```python
from build123d import *

# Parameters (mm, degrees)
SCHIZZO1_W                   = 63.34
SCHIZZO1_H                   = 103.98
ESTRUSIONE_ESTRUSIONE1_DEPTH = 4
SCHIZZO2_W                   = 63.34
SCHIZZO2_H                   = 103.98
SCHIZZO2_W_2                 = 53.34
SCHIZZO2_H_2                 = 93.98
ESTRUSIONE_ESTRUSIONE2_DEPTH = 35
FORO_PER_VITE_M2_1_D         = 2.4
SCHIZZO5_W                   = 33.34
SCHIZZO5_H                   = 15
TAGLIO_ESTRUSIONE1_DEPTH     = 126.106755432
TAGLIO_ESTRUSIONE2_DEPTH     = 132.87260726
RACCORDO1_R                  = 4


with BuildPart() as part:
    # Schizzo1 → Estrusione-Estrusione1 (new body)
    with BuildSketch(Plane(origin=(0, 0, 0), x_dir=(1, 0, 0), z_dir=(0, 1, 0))):
        with Locations((34.160538922, 55.414491018)):
            Rectangle(SCHIZZO1_W, SCHIZZO1_H)
    extrude(amount=ESTRUSIONE_ESTRUSIONE1_DEPTH)

    # Schizzo2 → Estrusione-Estrusione2 (add)
    with BuildSketch(Plane(origin=(0, 4, 0), x_dir=(1, 0, 0), z_dir=(0, 1, 0))):
        with Locations((34.160538922, 55.414491018)):
            Rectangle(SCHIZZO2_W, SCHIZZO2_H)
        with Locations((34.160538922, 55.414491018)):
            Rectangle(SCHIZZO2_W_2, SCHIZZO2_H_2, mode=Mode.SUBTRACT)
    extrude(amount=ESTRUSIONE_ESTRUSIONE2_DEPTH)

    # Foro per Vite M2-1 (through all)
    with Locations(Plane(origin=(0, 39, 0), x_dir=(1, 0, 0), z_dir=(0, 1, 0))):
        with Locations((4.990538922, 104.904491018), (63.330538922, 104.904491018), (63.330538922, 5.924491018), (4.990538922, 5.924491018)):
            Hole(FORO_PER_VITE_M2_1_D / 2)

    # Schizzo5 → Taglio-Estrusione1 (cut, through all)
    with BuildSketch(Plane.XY.offset(-102.404491018)):
        with Locations((34.160538922, 11.5)):
            Rectangle(SCHIZZO5_W, SCHIZZO5_H)
    extrude(amount=-TAGLIO_ESTRUSIONE1_DEPTH, mode=Mode.SUBTRACT)

    # Schizzo6 → Taglio-Estrusione2 (cut, through all)
    with BuildSketch(Plane(origin=(0, 0, 0), x_dir=(-1, 0, 0), z_dir=(0, -1, 0))):
        with BuildLine():
            Line((-31.160538922, 33.819804662), (-31.160538922, 20.424491018))
            ThreePointArc((-31.160538922, 20.424491018), (-31.74632536, 19.010277456), (-33.160538922, 18.424491018))
            Line((-33.160538922, 18.424491018), (-35.160538922, 18.424491018))
            ThreePointArc((-35.160538922, 18.424491018), (-36.574752485, 19.010277456), (-37.160538922, 20.424491018))
            Line((-37.160538922, 20.424491018), (-37.160538922, 33.819804662))
            ThreePointArc((-37.160538922, 33.819804662), (-37.632846353, 35.941125005), (-38.960538922, 37.661679204))
            ThreePointArc((-38.960538922, 37.661679204), (-34.160538922, 50.924491018), (-29.360538922, 37.661679204))
            ThreePointArc((-29.360538922, 37.661679204), (-30.688231491, 35.941125005), (-31.160538922, 33.819804662))
        make_face()
    extrude(amount=-TAGLIO_ESTRUSIONE2_DEPTH, mode=Mode.SUBTRACT)

    # Raccordo1
    raccordo1_edges = [part.edges().sort_by_distance(p)[0] for p in [
        (30.688231491, 4, -35.941125005),
        (31.160538922, 4, -27.12214784),
        (31.74632536, 4, -19.010277456),
        (34.160538922, 4, -18.424491018),
        (36.574752485, 4, -19.010277456),
        (37.160538922, 4, -27.12214784),
        (37.632846353, 4, -35.941125005),
        (34.160538922, 4, -50.924491018),
    ]]
    fillet(raccordo1_edges, radius=RACCORDO1_R - 0.0001)  # a hair under: the kernel refuses the full size


solid = part.part
```
Work out the finished part from the listing and answer in its coordinate system (mm). A direction names the side the tool comes from. Round coordinates to 2 decimals unless told otherwise and drop trailing zeros. Write each loop counter-clockwise with the first axis right and the second up, starting at its lowest first coordinate (ties: lowest second). Pieces come first, ordered by that corner, then holes. Notation, with made-up numbers: (-7.5, 79) -> (8.5, 79) arc R20 ccw to (8.5, 94) -> close; hole circle Ø9 at (-30.5, 40). An arc over 180 degrees is marked (long way). Write each question's results on one line, items separated by ' | '.
Q1. Determine the mould class of faces 1 (the flat face through (34, 0, -56)), 2 (the flat face through (34, 19, -3.424)), 3 (the flat face through (33.7, 19.2, -107.404)), 4 (the flat face through (34, 25, -102.404)) for opening direction Z: released by +Z, released by -Z, zero draft, split by the parting line, or undercut.
Data:
face 1: zero draft | face 2: released by +Z | face 3: released by -Z | face 4: undercut
Q2. Flat-ended cylindrical pins translate along their axes: P1, Ø1.9, axis at x = 4.99, z = -5.92, coming from the -Y side; P2, Ø17.5, axis at x = 34.16, z = -43.42, coming from the +Y side; P3, Ø1, axis at x = 43.5, z = -29.5, coming from the +Y side. Find the tip coordinate at first contact, or state that the pin passes through.
Data:
P1: through | P2: y = 2.91 | P3: y = 4
Q3. Section C-C, the plane y = 11 is taken. Write down the section's boundary in (x, z), then the cut area to 3 significant figures.
Data:
outline: (2.49, -107.4) -> (17.49, -107.4) -> (17.49, -102.4) -> (7.49, -102.4) -> (7.49, -8.42) -> (60.83, -8.42) -> (60.83, -102.4) -> (50.83, -102.4) -> (50.83, -107.4) -> (65.83, -107.4) -> (65.83, -3.42) -> (2.49, -3.42) -> close; hole circle Ø2.4 at (4.99, -104.9); hole circle Ø2.4 at (4.99, -5.92); hole circle Ø2.4 at (63.33, -104.9); hole circle Ø2.4 at (63.33, -5.92) | area: 1,390 mm^2
Q4. Section B-B, the plane x = 53.5 is taken. Write down the section's boundary in (y, z).
Data:
outline: (0, -107.4) -> (39, -107.4) -> (39, -102.4) -> (4, -102.4) -> (4, -8.42) -> (39, -8.42) -> (39, -3.42) -> (0, -3.42) -> close
Q5. Section D-D, the plane y = 34.5 is taken. Write down the section's boundary in (x, z).
Data:
outline: (2.49, -107.4) -> (65.83, -107.4) -> (65.83, -3.42) -> (2.49, -3.42) -> close; hole circle Ø2.4 at (4.99, -104.9); hole circle Ø2.4 at (4.99, -5.92); hole (7.49, -102.4) -> (60.83, -102.4) -> (60.83, -8.42) -> (7.49, -8.42) -> close; hole circle Ø2.4 at (63.33, -104.9); hole circle Ø2.4 at (63.33, -5.92)
Q6. Section A-A, the plane z = -12 is taken. Write down the section's boundary in (x, y).
Data:
outline: (2.49, 0) -> (65.83, 0) -> (65.83, 39) -> (60.83, 39) -> (60.83, 4) -> (7.49, 4) -> (7.49, 39) -> (2.49, 39) -> close
Q7. Straight lines are drawn through the part: line 1 along Z through (x, y) = (32.5, 33); line 2 along X through (y, z) = (12, -80.5); line 3 along Z through (x, y) = (6, 14). For each, find the intervals that lie inside material, in ascending order. Write a range as [from, to].
Data:
line 1: [-107.4, -102.4], [-8.42, -3.42] | line 2: [2.49, 7.49], [60.83, 65.83] | line 3: [-107.4, -105.55], [-104.26, -6.57], [-5.28, -3.42]
Q8. Which of the six approach directions +Z, -Z, +X, -X, +Y, -Y give full straight-line access (tool end or side, diameter ignored) to faces 5 (the cylindrical face through (4.44, 19.23, -4.86)), 6 (the flat face through (60.831, 21, -55)), 7 (the flat face through (17.491, 11, -105))?
Data:
face 5: +Y, -Y | face 6: +Y | face 7: -Z
